```python
from build123d import *

# Parameters (mm, degrees)
SKETCH1_R           = 2.1
BOSS_EXTRUDE1_DEPTH = 15


with BuildPart() as part:
    # Sketch1 → Boss-Extrude1 (new body)
    with BuildSketch(Plane.XY):
        with BuildLine():
            Line((-22.980970389, 18.03122292), (-19.621301934, 14.671554465))
            ThreePointArc((-19.621301934, 14.671554465), (-17.324116139, -17.324116139), (14.671554465, -19.621301934))
            Line((14.671554465, -19.621301934), (18.03122292, -22.980970389))
            ThreePointArc((18.03122292, -22.980970389), (22.980970389, -22.980970389), (22.980970389, -18.03122292))
            Line((22.980970389, -18.03122292), (19.621301934, -14.671554465))
            ThreePointArc((19.621301934, -14.671554465), (23.780652377, -5.893265015), (24.201713513, 3.811438449))
            ThreePointArc((24.201713513, 3.811438449), (24.731491872, 5.685176303), (26.5, 6.5))
            Line((26.5, 6.5), (26.5, 26.5))
            Line((26.5, 26.5), (6.014536774, 26.5))
            ThreePointArc((6.014536774, 26.5), (-4.885358384, 24.735246981), (-14.671554465, 19.621301934))
            Line((-14.671554465, 19.621301934), (-18.03122292, 22.980970389))
            ThreePointArc((-18.03122292, 22.980970389), (-22.980970389, 22.980970389), (-22.980970389, 18.03122292))
        make_face()
        with Locations((-20.506096654, 20.506096654)):
            Circle(SKETCH1_R, mode=Mode.SUBTRACT)
        with Locations((20.506096654, -20.506096654)):
            Circle(SKETCH1_R, mode=Mode.SUBTRACT)
    extrude(amount=BOSS_EXTRUDE1_DEPTH)


solid = part.part
```
Design review of the part built by this model. Coordinates are the model's own, in mm. A direction names the side the tool comes from. Give positions to 0.01 mm unless a question says otherwise; leave off trailing zeros. Write each loop counter-clockwise with the first axis right and the second up, starting at its lowest first coordinate (ties: lowest second). Pieces come first, ordered by that corner, then holes. Notation, with made-up numbers: (32.5, 88.25) - (55.5, 88.25) arc R28 ccw to (55.5, 122.25) - close; hole circle Ø5 at (1, 50.5). An arc over 180 degrees is marked (long way). Return JSON: item names as keys, results as strings. Group by question number.
(1) Mouldability with a two-part tool opening along Y and no side actions: class faces 6 (the cylindrical face through (-4.738, 24.784, 7.395)), 7 (the flat face through (16.33, -21.28, 7.4)), 8 (the flat face through (1, 1, 0)), 9 (the cylindrical face through (24.71, 5.66, 7.4)) as +Y half, -Y half, draft (parallel to the pull), parting line (faces both ways), or undercut.
(2) Insertion check: pin 1 (1.5 mm diameter, centred on y = -14, z = 9, fed in from -X); pin 2 (2 mm diameter, centred on x = -0.5, z = 9.5, fed in from +Y); pin 3 (1.5 mm diameter, centred on y = 21, z = 11, fed in from -X). Each pin has a flat end and moves straight along its axis. Give the tip position at first contact, or say it passes through.
(3) Machinability: for faces 1 (the flat face through (21.32, -16.37, 7.4)), 2 (the flat face through (-21.32, 16.37, 7.4)), 3 (the flat face through (-16.33, 21.28, 7.4)), 4 (the flat face through (26.5, 16, 7)), 5 (the cylindrical face through (-18.503, 21.137, 7.395)), which of the approach directions +Z, -Z, +X, -X, +Y, -Y give a long, thin tool a straight path to every point of the face, cutting with its end or side? Answer none if there is none.
(4) We need section B-B, the plane x = -20.5. Give the boundary of the cut face in (y, z).
(5) To check wall thickness, follow probe 1 along Y at (x, z) = (-22, 0.5); probe 2 along X at (y, z) = (21, 1.75) (3 decimals); probe 3 along Y at (x, z) = (-12.5, 12.25). State the ranges of each line that lie inside material, in increasing order.
(6) We need section D-D, the plane x = 7. Give the boundary of the cut face in (y, z).
(7) We need section C-C, the plane y = 2. Give the boundary of the cut face in (x, z), then the cut area to 3 significant figures.
(8) We need section A-A, the plane z = 4.5. Give the boundary of the cut face in (x, y), then the cut area to 3 significant figures.
Reported:
{
 "1": {"face 6": "+Y half", "face 7": "-Y half", "face 8": "draft", "face 9": "undercut"},
 "2": {"pin 1": "stops at x = -20.61", "pin 2": "stops at y = 26.06", "pin 3": "stops at x = -24.01"},
 "3": {"face 1": "+Z, -Z, +X", "face 2": "+Z, -Z, -X", "face 3": "+Z, -Z, +Y", "face 4": "+Z, -Z, +X, +Y, -Y", "face 5": "+Z, -Z"},
 "4": {"outline": "(-13.42, 0) - (13.42, 0) - (13.42, 15) - (-13.42, 15) - close; (15.55, 0) - (18.41, 0) - (18.41, 15) - (15.55, 15) - close; (22.61, 0) - (24.01, 0) - (24.01, 15) - (22.61, 15) - close"},
 "5": {"probe 1": "y = -10.78 to 10.78, 17.05 to 19.03, 21.98 to 23.67", "probe 2": "x = -23.971 to -22.547, -18.465 to -16.05, -12.687 to 26.5", "probe 3": "y = -21.07 to 21.12"},
 "6": {"outline": "(-23.48, 0) - (26.5, 0) - (26.5, 15) - (-23.48, 15) - close"},
 "7": {"outline": "(-24.42, 0) - (24.42, 0) - (24.42, 15) - (-24.42, 15) - close", "area": "733 mm2"},
 "8": {"outline": "(-22.98, 18.03) - (-19.62, 14.67) arc R24.5 ccw to (14.67, -19.62) - (18.03, -22.98) arc R3.5 ccw to (22.98, -18.03) - (19.62, -14.67) arc R24.5 ccw to (24.2, 3.81) arc R2.33 cw to (26.5, 6.5) - (26.5, 26.5) - (6.01, 26.5) arc R34.54 ccw to (-14.67, 19.62) - (-18.03, 22.98) arc R3.5 ccw to start; hole circle Ø4.2 at (-20.51, 20.51); hole circle Ø4.2 at (20.51, -20.51)", "area": "2,190 mm2"}
}
